Here's the drawing with two shaded views (mm, measured from the low corner). I have some questions. Give positions to 0.01 mm unless a question says otherwise; leave off trailing zeros. Loops run counter-clockwise (first coordinate to the right, second up) from the corner with the lowest first, then second, coordinate; pieces in that order, holes last.
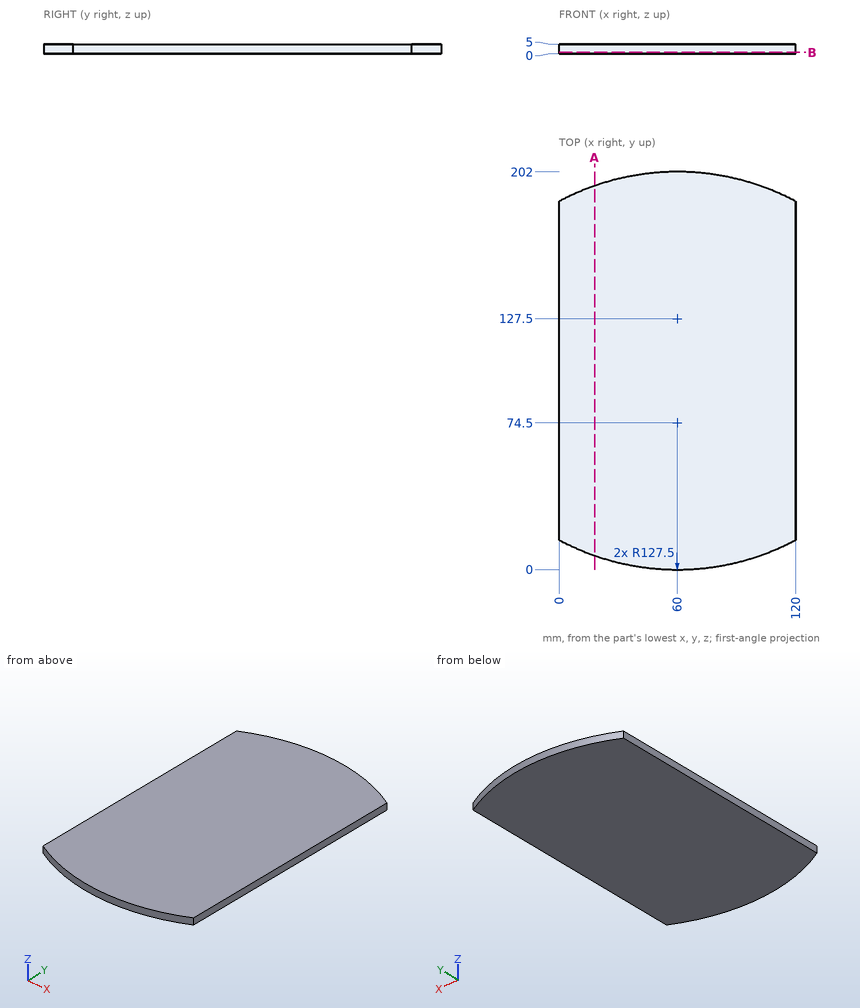
(1) Please list where these lines run through material, in increasing order: probe 1 along Y at (x, z) = (61.5, 3.4); probe 2 along Y at (x, z) = (18.5, 0.9); probe 3 along X at (y, z) = (193, 1.35).
Returned:
probe 1: y = 0.01 to 201.99
probe 2: y = 6.94 to 195.06
probe 3: x = 12.95 to 107.05
(2) Will these pins go through, and if not, where does the flat tip stop? P1, Ø2, axis at x = 83, z = 1, coming from the -Y side; P2, Ø3, axis at x = 43, z = 4, coming from the -Y side.
Returned:
P1: stops at y = 1.91
P2: stops at y = 0.95
(3) Suppose I cut it at A-A on x = 18. List the corners of the cut face in (y, z) for me.
Returned:
outline: (7.12, 0) - (194.88, 0) - (194.88, 5) - (7.12, 5) - close
(4) Suppose I cut it at B-B on z = 0.75. List the corners of the cut face in (x, y) for me, plus the area to 3 significant figures.
Returned:
outline: (0, 15) arc R127.5 ccw to (120, 15) - (120, 187) arc R127.5 ccw to (0, 187) - close
area: 23,100 mm2
